```python
from build123d import *

# Parameters (mm, degrees)
BOSS_EXTRUDE1_DEPTH = 31.75
SKETCH2_R           = 3.175
CUT_EXTRUDE1_DEPTH  = 19.05
CHAMFER1_SIZE       = 7.874
SKETCH3_R           = 2.1828125
CUT_EXTRUDE2_DEPTH  = 19.05
CHAMFER2_SIZE       = 7.874
CHAMFER3_SIZE       = 0.254


with BuildPart() as part:
    # Sketch1 → Boss-Extrude1 (new body)
    with BuildSketch(Plane(origin=(0, 0, 0), x_dir=(0, 0, -1), z_dir=(1, 0, 0))):
        Polygon((0, 0), (0, 44.45), (-6.35, 44.45), (-6.35, 25.4), (-76.2, 25.4), (-76.2, 19.05), (-6.35, 19.05), (-6.35, 0), align=None)
    extrude(amount=BOSS_EXTRUDE1_DEPTH)

    # Sketch2 → Cut-Extrude1 (cut)
    with BuildSketch(Plane.XY.offset(6.35)):
        with Locations((6.35, 38.1)):
            Circle(SKETCH2_R)
        with Locations((25.4, 38.1)):
            Circle(SKETCH2_R)
        with Locations((6.35, 6.35)):
            Circle(SKETCH2_R)
        with Locations((25.4, 6.35)):
            Circle(SKETCH2_R)
    extrude(amount=-CUT_EXTRUDE1_DEPTH, mode=Mode.SUBTRACT)

    # Chamfer1
    chamfer1_edges = [part.edges().sort_by_distance(p)[0] for p in [
        (15.875, 19.05, 6.35),
        (15.875, 25.4, 6.35),
    ]]
    chamfer(chamfer1_edges, length=CHAMFER1_SIZE)

    # Sketch3 → Cut-Extrude2 (cut)
    with BuildSketch(Plane(origin=(0, 25.4, 0), x_dir=(1, 0, 0), z_dir=(0, 1, 0))):
        with Locations(Location((15.875, -69.85, 0), (0, 0, 270))):
            Circle(SKETCH3_R)
        with Locations(Location((15.875, -31.75, 0), (0, 0, 270))):
            Circle(SKETCH3_R)
    extrude(amount=-CUT_EXTRUDE2_DEPTH, mode=Mode.SUBTRACT)

    # Chamfer2
    chamfer2_edges = [part.edges().sort_by_distance(p)[0] for p in [
        (31.75, 22.225, 76.2),
        (0, 22.225, 76.2),
    ]]
    chamfer(chamfer2_edges, length=CHAMFER2_SIZE)

    # Chamfer3
    chamfer3_edges = [part.edges().sort_by_distance(p)[0] for p in [
        (0, 22.225, 0),
        (15.875, 44.45, 0),
        (15.875, 0, 0),
        (22.225, 38.1, 0),
        (3.175, 6.35, 0),
        (22.225, 6.35, 0),
        (3.175, 38.1, 0),
        (31.75, 22.225, 0),
    ]]
    chamfer(chamfer3_edges, length=CHAMFER3_SIZE)


solid = part.part
```
Model file for the job. Use its own axes, mm. A direction names the side the tool comes from. Give positions to 0.01 mm unless a question says otherwise; leave off trailing zeros. Write each loop counter-clockwise with the first axis right and the second up, starting at its lowest first coordinate (ties: lowest second). Pieces come first, ordered by that corner, then holes. Notation, with made-up numbers: (87, 53.5) - (127, 53.5) arc R17 cw to (127, 62.5) - close; hole circle Ø6 at (14, -25.5). An arc over 180 degrees is marked (long way). One line per question, with ' | ' between items. Start each with the question number.
(1) 3-axis set-ups, long thin cutter, end or side, ignore diameter. For faces 1 (the face through (27.868, 22.269, 72.208)), 2 (the face through (16, 25.4, 45)), 3 (the face through (16, 6, 6.35)): which of +Z, -Z, +X, -X, +Y, -Y reach the whole face in a straight line?
(2) Slice it at A-A on y = 38.1. Write the cut outline in (x, z) (3 decimals), plus the area to 3 significant figures.
(3) Slice it at D-D on x = 6.35. Write the cut outline in (y, z) (3 decimals), plus the area to 3 significant figures.
(4) Wall check: line 1 along Y through (x, z) = (6.35, 5) (3 decimals); line 2 along X through (y, z) = (5, 6); line 3 along Y through (x, z) = (26, 47.5). Give the ranges that are in metal, low to high. Write a range as from..to.
(5) Pin check, flat tips, straight feed: P1, Ø2, axis at x = 22, y = 13.5, coming from the +Z side; P2, Ø12, axis at y = 8.5, z = 59, coming from the -X side; P3, Ø6, axis at x = 24, y = 9, coming from the +Z side; P4, Ø5.5, axis at x = 22, y = 5, coming from the +Z side. Stop position of each tip, or through.
(6) Two-plate mould, pull along Z, no slides. Class faces 4 (the face through (15.97, 22.27, 29.57)), 5 (the face through (14.547, 22.269, 68.118)), 6 (the face through (16, 19.05, 46)), 7 (the face through (16, 39, 6.35)): +Z half, -Z half, draft (parallel to the pull), parting line (faces both ways), or undercut.
(7) Slice it at C-C on y = 21. Write the cut outline in (x, z) (3 decimals).
(8) Slice it at B-B on z = 31.75. Write the cut outline in (x, y).
Results below:
1) face 1: +Z, +X, +Y, -Y | face 2: +Z, +X, -X, +Y | face 3: +Z, +X, -X, -Y
2) outline: (0, 0.254) - (0.254, 0) - (2.921, 0) - (3.175, 0.254) - (3.175, 6.35) - (0, 6.35) - close; (9.525, 0.254) - (9.779, 0) - (21.971, 0) - (22.225, 0.254) - (22.225, 6.35) - (9.525, 6.35) - close; (28.575, 0.254) - (28.829, 0) - (31.496, 0) - (31.75, 0.254) - (31.75, 6.35) - (28.575, 6.35) - close | area: 121 mm^2
3) outline: (0, 0.254) - (0.254, 0) - (2.921, 0) - (3.175, 0.254) - (3.175, 6.35) - (0, 6.35) - close; (9.525, 0.254) - (9.779, 0) - (34.671, 0) - (34.925, 0.254) - (34.925, 6.35) - (33.274, 6.35) - (25.4, 14.224) - (25.4, 74.676) - (19.05, 74.676) - (19.05, 14.224) - (11.176, 6.35) - (9.525, 6.35) - close; (41.275, 0.254) - (41.529, 0) - (44.196, 0) - (44.45, 0.254) - (44.45, 6.35) - (41.275, 6.35) - close | area: 697 mm^2
4) line 1: 0..3.175, 9.525..34.925, 41.275..44.45 | line 2: 0..3.48, 9.22..22.53, 28.27..31.75 | line 3: 19.05..25.4
5) P1: z = 9.67 | P2: through | P3: z = 7.17 | P4: z = 6.35
6) face 4: undercut | face 5: undercut | face 6: draft | face 7: +Z half
7) outline: (0, 0.254) - (0.254, 0) - (31.496, 0) - (31.75, 0.254) - (31.75, 68.326) - (23.876, 76.2) - (7.874, 76.2) - (0, 68.326) - close; hole circle Ø4.366 at (15.875, 31.75); hole circle Ø4.366 at (15.875, 69.85)
8) outline: (0, 19.05) - (13.69, 19.05) - (13.69, 25.4) - (0, 25.4) - close; (18.06, 19.05) - (31.75, 19.05) - (31.75, 25.4) - (18.06, 25.4) - close
